CAD build for the part. Positions are in the model's coordinates, mm. A direction names the side the tool comes from. Give positions to 0.01 mm unless a question says otherwise; leave off trailing zeros. Order: outer loops, then holes, each group sorted by start corner. A loop starts at its lowest first (then second) coordinate and runs counter-clockwise, first axis right, second up.
```python
from build123d import *

# Parameters (mm, degrees)
F1_DEPTH = 6


# Not quite as in the source:
# - a feature names something its author has since deleted; it is built from what else it names


with BuildPart() as f1:
    # F0 (on Top) → F1 (new body)
    with BuildSketch(Plane.XY):
        with BuildLine():
            Line((19.975, -0.9996874512), (20, 0))
            Line((20, 0), (19.975, 0.9996874512))
            ThreePointArc((19.975, 0.9996874512), (19.6961550602, 3.4729635533), (19.1122733455, 5.892453442))
            Line((19.1122733455, 5.892453442), (18.7938524157, 6.8404028665))
            Line((18.7938524157, 6.8404028665), (18.4284468549, 7.7712512839))
            ThreePointArc((18.4284468549, 7.7712512839), (17.3205080757, 10), (15.9443244585, 12.0738774867))
            Line((15.9443244585, 12.0738774867), (15.3208888624, 12.8557521937))
            Line((15.3208888624, 12.8557521937), (14.6591510441, 13.6054875203))
            ThreePointArc((14.6591510441, 13.6054875203), (12.8557521937, 15.3208888624), (10.8532547285, 16.799013715))
            Line((10.8532547285, 16.799013715), (10, 17.3205080757))
            Line((10, 17.3205080757), (9.1217452715, 17.7987011662))
            ThreePointArc((9.1217452715, 17.7987011662), (6.8404028665, 18.7938524157), (4.4531223014, 19.4979409623))
            Line((4.4531223014, 19.4979409623), (3.4729635533, 19.6961550602))
            Line((3.4729635533, 19.6961550602), (2.4841223964, 19.8451287705))
            ThreePointArc((2.4841223964, 19.8451287705), (0, 20), (-2.4841223964, 19.8451287705))
            Line((-2.4841223964, 19.8451287705), (-3.4729635533, 19.6961550602))
            Line((-3.4729635533, 19.6961550602), (-4.4531223014, 19.4979409623))
            ThreePointArc((-4.4531223014, 19.4979409623), (-6.8404028665, 18.7938524157), (-9.1217452715, 17.7987011662))
            Line((-9.1217452715, 17.7987011662), (-10, 17.3205080757))
            Line((-10, 17.3205080757), (-10.8532547285, 16.799013715))
            ThreePointArc((-10.8532547285, 16.799013715), (-12.8557521937, 15.3208888624), (-14.6591510441, 13.6054875203))
            Line((-14.6591510441, 13.6054875203), (-15.3208888624, 12.8557521937))
            Line((-15.3208888624, 12.8557521937), (-15.9443244585, 12.0738774867))
            ThreePointArc((-15.9443244585, 12.0738774867), (-17.3205080757, 10), (-18.4284468549, 7.7712512839))
            Line((-18.4284468549, 7.7712512839), (-18.7938524157, 6.8404028665))
            Line((-18.7938524157, 6.8404028665), (-19.1122733455, 5.892453442))
            ThreePointArc((-19.1122733455, 5.892453442), (-19.6961550602, 3.4729635533), (-19.975, 0.9996874512))
            Line((-19.975, 0.9996874512), (-20, 0))
            Line((-20, 0), (-19.975, -0.9996874512))
            ThreePointArc((-19.975, -0.9996874512), (-19.6961550602, -3.4729635533), (-19.1122733455, -5.892453442))
            Line((-19.1122733455, -5.892453442), (-18.7938524157, -6.8404028665))
            Line((-18.7938524157, -6.8404028665), (-18.4284468549, -7.7712512839))
            ThreePointArc((-18.4284468549, -7.7712512839), (-17.3205080757, -10), (-15.9443244585, -12.0738774867))
            Line((-15.9443244585, -12.0738774867), (-15.3208888624, -12.8557521937))
            Line((-15.3208888624, -12.8557521937), (-14.6591510441, -13.6054875203))
            ThreePointArc((-14.6591510441, -13.6054875203), (-12.8557521937, -15.3208888624), (-10.8532547285, -16.799013715))
            Line((-10.8532547285, -16.799013715), (-10, -17.3205080757))
            Line((-10, -17.3205080757), (-9.1217452715, -17.7987011662))
            ThreePointArc((-9.1217452715, -17.7987011662), (-6.8404028665, -18.7938524157), (-4.4531223014, -19.4979409623))
            Line((-4.4531223014, -19.4979409623), (-3.4729635533, -19.6961550602))
            Line((-3.4729635533, -19.6961550602), (-2.4841223964, -19.8451287705))
            ThreePointArc((-2.4841223964, -19.8451287705), (0, -20), (2.4841223964, -19.8451287705))
            Line((2.4841223964, -19.8451287705), (3.4729635533, -19.6961550602))
            Line((3.4729635533, -19.6961550602), (4.4531223014, -19.4979409623))
            ThreePointArc((4.4531223014, -19.4979409623), (6.8404028665, -18.7938524157), (9.1217452715, -17.7987011662))
            Line((9.1217452715, -17.7987011662), (10, -17.3205080757))
            Line((10, -17.3205080757), (10.8532547285, -16.799013715))
            ThreePointArc((10.8532547285, -16.799013715), (12.8557521937, -15.3208888624), (14.6591510441, -13.6054875203))
            Line((14.6591510441, -13.6054875203), (15.3208888624, -12.8557521937))
            Line((15.3208888624, -12.8557521937), (15.9443244585, -12.0738774867))
            ThreePointArc((15.9443244585, -12.0738774867), (17.3205080757, -10), (18.4284468549, -7.7712512839))
            Line((18.4284468549, -7.7712512839), (18.7938524157, -6.8404028665))
            Line((18.7938524157, -6.8404028665), (19.1122733455, -5.892453442))
            ThreePointArc((19.1122733455, -5.892453442), (19.6961550602, -3.4729635533), (19.975, -0.9996874512))
        make_face()
        with BuildLine():
            ThreePointArc((-2.4841223964, 19.8451287705), (0, 20), (2.4841223964, 19.8451287705))
            Line((2.4841223964, 19.8451287705), (1, 24))
            Line((1, 24), (0, 24))
            Line((0, 24), (-1, 24))
            Line((-1, 24), (-2.4841223964, 19.8451287705))
        make_face()
        with BuildLine():
            ThreePointArc((4.4531223014, 19.4979409623), (6.8404028665, 18.7938524157), (9.1217452715, 17.7987011662))
            Line((9.1217452715, 17.7987011662), (9.1481760606, 22.2106027555))
            Line((9.1481760606, 22.2106027555), (8.2084834398, 22.5526228989))
            Line((8.2084834398, 22.5526228989), (7.268790819, 22.8946430422))
            Line((7.268790819, 22.8946430422), (4.4531223014, 19.4979409623))
        make_face()
        with BuildLine():
            ThreePointArc((10.8532547285, 16.799013715), (12.8557521937, 15.3208888624), (14.6591510441, 13.6054875203))
            Line((14.6591510441, 13.6054875203), (16.1929470756, 17.7422790252))
            Line((16.1929470756, 17.7422790252), (15.4269026325, 18.3850666349))
            Line((15.4269026325, 18.3850666349), (14.6608581894, 19.0278542445))
            Line((14.6608581894, 19.0278542445), (10.8532547285, 16.799013715))
        make_face()
        with BuildLine():
            ThreePointArc((15.9443244585, 12.0738774867), (17.3205080757, 10), (18.4284468549, 7.7712512839))
            Line((18.4284468549, 7.7712512839), (21.2846096908, 11.1339745962))
            Line((21.2846096908, 11.1339745962), (20.7846096908, 12))
            Line((20.7846096908, 12), (20.2846096908, 12.8660254038))
            Line((20.2846096908, 12.8660254038), (15.9443244585, 12.0738774867))
        make_face()
        with BuildLine():
            ThreePointArc((19.1122733455, 5.892453442), (19.6961550602, 3.4729635533), (19.975, 0.9996874512))
            Line((19.975, 0.9996874512), (23.80903425, 3.182748511))
            Line((23.80903425, 3.182748511), (23.6353860723, 4.167556264))
            Line((23.6353860723, 4.167556264), (23.4617378946, 5.152364017))
            Line((23.4617378946, 5.152364017), (19.1122733455, 5.892453442))
        make_face()
        with BuildLine():
            Line((23.80903425, -3.182748511), (19.975, -0.9996874512))
            ThreePointArc((19.975, -0.9996874512), (19.6961550602, -3.4729635533), (19.1122733455, -5.892453442))
            Line((19.1122733455, -5.892453442), (23.4617378946, -5.152364017))
            Line((23.4617378946, -5.152364017), (23.6353860723, -4.167556264))
            Line((23.6353860723, -4.167556264), (23.80903425, -3.182748511))
        make_face()
        with BuildLine():
            Line((21.2846096908, -11.1339745962), (18.4284468549, -7.7712512839))
            ThreePointArc((18.4284468549, -7.7712512839), (17.3205080757, -10), (15.9443244585, -12.0738774867))
            Line((15.9443244585, -12.0738774867), (20.2846096908, -12.8660254038))
            Line((20.2846096908, -12.8660254038), (20.7846096908, -12))
            Line((20.7846096908, -12), (21.2846096908, -11.1339745962))
        make_face()
        with BuildLine():
            Line((16.1929470756, -17.7422790252), (14.6591510441, -13.6054875203))
            ThreePointArc((14.6591510441, -13.6054875203), (12.8557521937, -15.3208888624), (10.8532547285, -16.799013715))
            Line((10.8532547285, -16.799013715), (14.6608581894, -19.0278542445))
            Line((14.6608581894, -19.0278542445), (15.4269026325, -18.3850666349))
            Line((15.4269026325, -18.3850666349), (16.1929470756, -17.7422790252))
        make_face()
        with BuildLine():
            Line((9.1481760606, -22.2106027555), (9.1217452715, -17.7987011662))
            ThreePointArc((9.1217452715, -17.7987011662), (6.8404028665, -18.7938524157), (4.4531223014, -19.4979409623))
            Line((4.4531223014, -19.4979409623), (7.268790819, -22.8946430422))
            Line((7.268790819, -22.8946430422), (8.2084834398, -22.5526228989))
            Line((8.2084834398, -22.5526228989), (9.1481760606, -22.2106027555))
        make_face()
        with BuildLine():
            Line((1, -24), (2.4841223964, -19.8451287705))
            ThreePointArc((2.4841223964, -19.8451287705), (0, -20), (-2.4841223964, -19.8451287705))
            Line((-2.4841223964, -19.8451287705), (-1, -24))
            Line((-1, -24), (0, -24))
            Line((0, -24), (1, -24))
        make_face()
        with BuildLine():
            Line((-7.268790819, -22.8946430422), (-4.4531223014, -19.4979409623))
            ThreePointArc((-4.4531223014, -19.4979409623), (-6.8404028665, -18.7938524157), (-9.1217452715, -17.7987011662))
            Line((-9.1217452715, -17.7987011662), (-9.1481760606, -22.2106027555))
            Line((-9.1481760606, -22.2106027555), (-8.2084834398, -22.5526228989))
            Line((-8.2084834398, -22.5526228989), (-7.268790819, -22.8946430422))
        make_face()
        with BuildLine():
            Line((-14.6608581894, -19.0278542445), (-10.8532547285, -16.799013715))
            ThreePointArc((-10.8532547285, -16.799013715), (-12.8557521937, -15.3208888624), (-14.6591510441, -13.6054875203))
            Line((-14.6591510441, -13.6054875203), (-16.1929470756, -17.7422790252))
            Line((-16.1929470756, -17.7422790252), (-15.4269026325, -18.3850666349))
            Line((-15.4269026325, -18.3850666349), (-14.6608581894, -19.0278542445))
        make_face()
        with BuildLine():
            Line((-20.2846096908, -12.8660254038), (-15.9443244585, -12.0738774867))
            ThreePointArc((-15.9443244585, -12.0738774867), (-17.3205080757, -10), (-18.4284468549, -7.7712512839))
            Line((-18.4284468549, -7.7712512839), (-21.2846096908, -11.1339745962))
            Line((-21.2846096908, -11.1339745962), (-20.7846096908, -12))
            Line((-20.7846096908, -12), (-20.2846096908, -12.8660254038))
        make_face()
        with BuildLine():
            Line((-23.4617378946, -5.152364017), (-19.1122733455, -5.892453442))
            ThreePointArc((-19.1122733455, -5.892453442), (-19.6961550602, -3.4729635533), (-19.975, -0.9996874512))
            Line((-19.975, -0.9996874512), (-23.80903425, -3.182748511))
            Line((-23.80903425, -3.182748511), (-23.6353860723, -4.167556264))
            Line((-23.6353860723, -4.167556264), (-23.4617378946, -5.152364017))
        make_face()
        with BuildLine():
            ThreePointArc((-19.975, 0.9996874512), (-19.6961550602, 3.4729635533), (-19.1122733455, 5.892453442))
            Line((-19.1122733455, 5.892453442), (-23.4617378946, 5.152364017))
            Line((-23.4617378946, 5.152364017), (-23.6353860723, 4.167556264))
            Line((-23.6353860723, 4.167556264), (-23.80903425, 3.182748511))
            Line((-23.80903425, 3.182748511), (-19.975, 0.9996874512))
        make_face()
        with BuildLine():
            ThreePointArc((-18.4284468549, 7.7712512839), (-17.3205080757, 10), (-15.9443244585, 12.0738774867))
            Line((-15.9443244585, 12.0738774867), (-20.2846096908, 12.8660254038))
            Line((-20.2846096908, 12.8660254038), (-20.7846096908, 12))
            Line((-20.7846096908, 12), (-21.2846096908, 11.1339745962))
            Line((-21.2846096908, 11.1339745962), (-18.4284468549, 7.7712512839))
        make_face()
        with BuildLine():
            ThreePointArc((-14.6591510441, 13.6054875203), (-12.8557521937, 15.3208888624), (-10.8532547285, 16.799013715))
            Line((-10.8532547285, 16.799013715), (-14.6608581894, 19.0278542445))
            Line((-14.6608581894, 19.0278542445), (-15.4269026325, 18.3850666349))
            Line((-15.4269026325, 18.3850666349), (-16.1929470756, 17.7422790252))
            Line((-16.1929470756, 17.7422790252), (-14.6591510441, 13.6054875203))
        make_face()
        with BuildLine():
            ThreePointArc((-9.1217452715, 17.7987011662), (-6.8404028665, 18.7938524157), (-4.4531223014, 19.4979409623))
            Line((-4.4531223014, 19.4979409623), (-7.268790819, 22.8946430422))
            Line((-7.268790819, 22.8946430422), (-8.2084834398, 22.5526228989))
            Line((-8.2084834398, 22.5526228989), (-9.1481760606, 22.2106027555))
            Line((-9.1481760606, 22.2106027555), (-9.1217452715, 17.7987011662))
        make_face()
    extrude(amount=F1_DEPTH)


solid = f1.part
```
Item 1: Drop a flat-ended pin along its axis: pin 1 Ø6 at (x, y) = (18, 17) entering from +Z. Give the stop position or say it passes through.
Item 2: Two-plate mould, pull along X, no slides. Class faces 5 (the face through (-12.73, 17.898, 2.958)), 6 (the face through (-15.437, 15.703, 2.958)), 7 (the face through (21.317, 5.517, 2.958)): released by +X, released by -X, zero draft, split by the parting line, or undercut.
Item 3: Slice it at A-A (y = -21). Give the cut face in (x, z), and give its area (3 significant figures).
Item 4: Wall check: L1, parallel to X at y = 17.5, z = 0.5; L2, parallel to X at y = 18, z = 5.55; L3, parallel to Y at x = 10, z = 4.6. Give the ranges that are in metal, low to high.
Item 5: Tool access for faces 1 (the face through (12.784, 17.929, 2.958)), 2 (the face through (1.732, -21.952, 2.958)), 3 (the face through (15.437, -15.703, 2.958)), 4 (the face through (-19.88, 9.48, 2.96)): list every direction of +Z, -Z, +X, -X, +Y, -Y with a clear straight run to the whole face (end or side of a thin tool).
Item 6: Slice it at B-B (x = -14). Give the cut face in (y, z).
Item 7: Slice it at C-C (y = 14.5). Give the cut face in (x, z), and give its area (3 significant figures).
A:
1. pin 1: stops at z = 6
2. face 5: undercut
2. face 6: released by -X
2. face 7: released by +X
3. outline: (-9.14, 0) - (-5.7, 0) - (-5.7, 6) - (-9.14, 6) - close; (-2.07, 0) - (2.07, 0) - (2.07, 6) - (-2.07, 6) - close; (5.7, 0) - (9.14, 0) - (9.14, 6) - (5.7, 6) - close
3. area: 66.2 mm2
4. L1: x = -16.1 to -12.05, -9.67 to 9.67, 12.05 to 16.1
4. L2: x = -15.89 to -12.9, -9.12 to 9.12, 12.9 to 15.89
4. L3: y = -17.32 to 17.32
5. face 1: +Z, -Z, +Y
5. face 2: +Z, -Z, -Y
5. face 3: +Z, -Z, +X
5. face 4: +Z, -Z, -X
6. outline: (-18.64, 0) - (18.64, 0) - (18.64, 6) - (-18.64, 6) - close
7. outline: (-14.99, 0) - (14.99, 0) - (14.99, 6) - (-14.99, 6) - close
7. area: 180 mm2
